Could you check a few things on this model? Use its own coordinates, in mm. Face numbers are marked on the shaded views. A direction names the side the tool comes from. Round coordinates to 2 decimals unless told otherwise and drop trailing zeros. Loops run counter-clockwise (first coordinate to the right, second up) from the corner with the lowest first, then second, coordinate; pieces in that order, holes last. Notation, with made-up numbers: (83.25, 59.25) -> (99.25, 59.25) arc R19 cw to (99.25, 91.25) -> close; hole circle Ø11 at (75.5, -38.5). An arc over 180 degrees is marked (long way). Put each result on its own line as item: value. Start each with the question number.
1. I need wall thicknesses on line 1 (X direction, y = -44, z = 19); line 2 (X direction, y = -45.5, z = 37.5); line 3 (Y direction, x = -33, z = 30). Which ranges of each line are inside material? Lowest first, please. Write a range as [from, to].
2. Which directions (+Z, -Z, +X, -X, +Y, -Y) give clear straight access to the entire face, cutting with the end or side of a thin tool? Please do the marked faces 1 and 2.
3. Imagine slicing it at A-A, the plane y = -23.5. Please give me the cut outline in (x, z), and give its area (3 significant figures).
4. Imagine slicing it at C-C, the plane z = 27. Please give me the cut outline in (x, y), and give its area (3 significant figures).
5. I'm going to push flat-ended pins straight in: P1, Ø3, axis at x = 21.5, z = 27, coming from the -Y side; P2, Ø1, axis at y = -41, z = 48.5, coming from the +X side; P3, Ø2, axis at y = -16.5, z = 27.5, coming from the +X side. Where does each tip first touch, or does it pass through?
6. Imagine slicing it at D-D, the plane y = -9. Please give me the cut outline in (x, z), and give its area (3 significant figures).
7. If we mould it in two halves opening along X, with no side actions, what happens to the marked faces 3, 4 and 5? For each: pulls with the +X half, pulls with the -X half, needs draft (parallel to the pull), parting line crosses it, or undercut.
8. Imagine slicing it at B-B, the plane x = -43.5. Please give me the cut outline in (y, z), and give its area (3 significant figures).
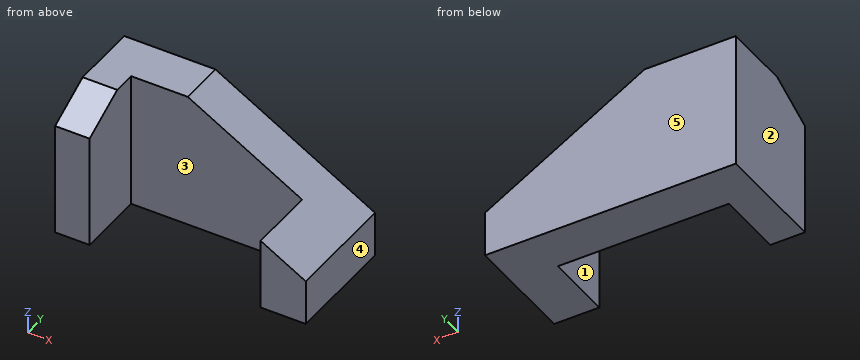
```python
from build123d import *

# Parameters (mm, degrees)
F1_DEPTH = 50
F2_W     = 75
F2_H     = 30
F3_DEPTH = 60
F5_DEPTH = 56


with BuildPart() as f1:
    # F0 (on Front) → F1 (new body)
    with BuildSketch(Plane.XZ):
        Polygon((-55.158045, 60), (-55.158045, 0), (54.841955, 0), (54.841955, 20), (-15.158045, 60), align=None)
    extrude(amount=F1_DEPTH)

    # F2 (on Top) → F3 (cut)
    with BuildSketch(Plane.XY):
        with Locations((-2.5, -35)):
            Rectangle(F2_W, F2_H)
    extrude(amount=F3_DEPTH, mode=Mode.SUBTRACT)

    # F4 (on Right) → F5 (cut, symmetric)
    with BuildSketch(Plane.YZ):
        Polygon((-50, 50), (-30, 60), (-50, 60), align=None)
    extrude(amount=F5_DEPTH, both=True, mode=Mode.SUBTRACT)


solid = f1.part
```
Entries:
1. line 1: [-55.16, -40], [35, 54.84]
1. line 2: [-55.16, -40]
1. line 3: [-20, 0]
2. face 1: +Z, -Z, -Y
2. face 2: +Z, -Z, -X, +Y, -Y
3. outline: (-55.16, 0) -> (-40, 0) -> (-40, 60) -> (-55.16, 60) -> close; (35, 0) -> (54.84, 0) -> (54.84, 20) -> (35, 31.34) -> close
3. area: 1,420 mm^2
4. outline: (-55.16, -50) -> (-40, -50) -> (-40, -20) -> (35, -20) -> (35, -50) -> (42.59, -50) -> (42.59, 0) -> (-55.16, 0) -> close
4. area: 2,640 mm^2
5. P1: y = -20
5. P2: x = -40
5. P3: x = 43.47
6. outline: (-55.16, 0) -> (54.84, 0) -> (54.84, 20) -> (-15.16, 60) -> (-55.16, 60) -> close
6. area: 5,200 mm^2
7. face 3: undercut
7. face 4: pulls with the +X half
7. face 5: needs draft
8. outline: (-50, 0) -> (0, 0) -> (0, 60) -> (-30, 60) -> (-50, 50) -> close
8. area: 2,900 mm^2
